The figure shows three views and two pictorial views of one solid part (mm, origin at its lowest corner). Answer the questions. A direction names the side the tool comes from. Coordinates: 2 decimals unless noted, no trailing zeros. Loops run counter-clockwise (first coordinate to the right, second up) from the corner with the lowest first, then second, coordinate; pieces in that order, holes last. Notation, with made-up numbers: (45.5, -11.75) -> (64.5, -11.75) arc R30 ccw to (64.5, 19.25) -> close; hole circle Ø1 at (43.5, -37.5). An arc over 180 degrees is marked (long way). Answer as a JSON object with one key per item and string values. Group by question number.
1) Determine the mould class of the marked faces 3, 4 and 5 for opening direction Y: released by +Y, released by -Y, zero draft, split by the parting line, or undercut.
2) Section C-C, the plane x = 3.5 is taken. Give the vertices of the cut face in (y, z).
3) Section A-A, the plane y = 6 is taken. Give the vertices of the cut face in (x, z).
4) Consider probe 1 along X at (y, z) = (5.75, 5.3); probe 2 along Y at (x, z) = (2.5, 1); probe 3 along X at (y, z) = (6.75, 5.3). Determine where each line is inside the solid, lowest interval first. Write a range as [from, to].
5) A flat-ended cylindrical pin translates along its axis: P1, Ø1.2, axis at x = 3.5, z = 1.5, coming from the +Y side. Find the tip coordinate at first contact, or state that the pin passes through.
6) Section D-D, the plane y = 7.75 is taken. Give the vertices of the cut face in (x, z), plus the area to 3 significant figures.
7) Which of the six approach directions +Z, -Z, +X, -X, +Y, -Y give full straight-line access (tool end or side, diameter ignored) to the marked faces 1 and 2?
8) Section B-B, the plane z = 1.7 is taken. Give the vertices of the cut face in (x, y).
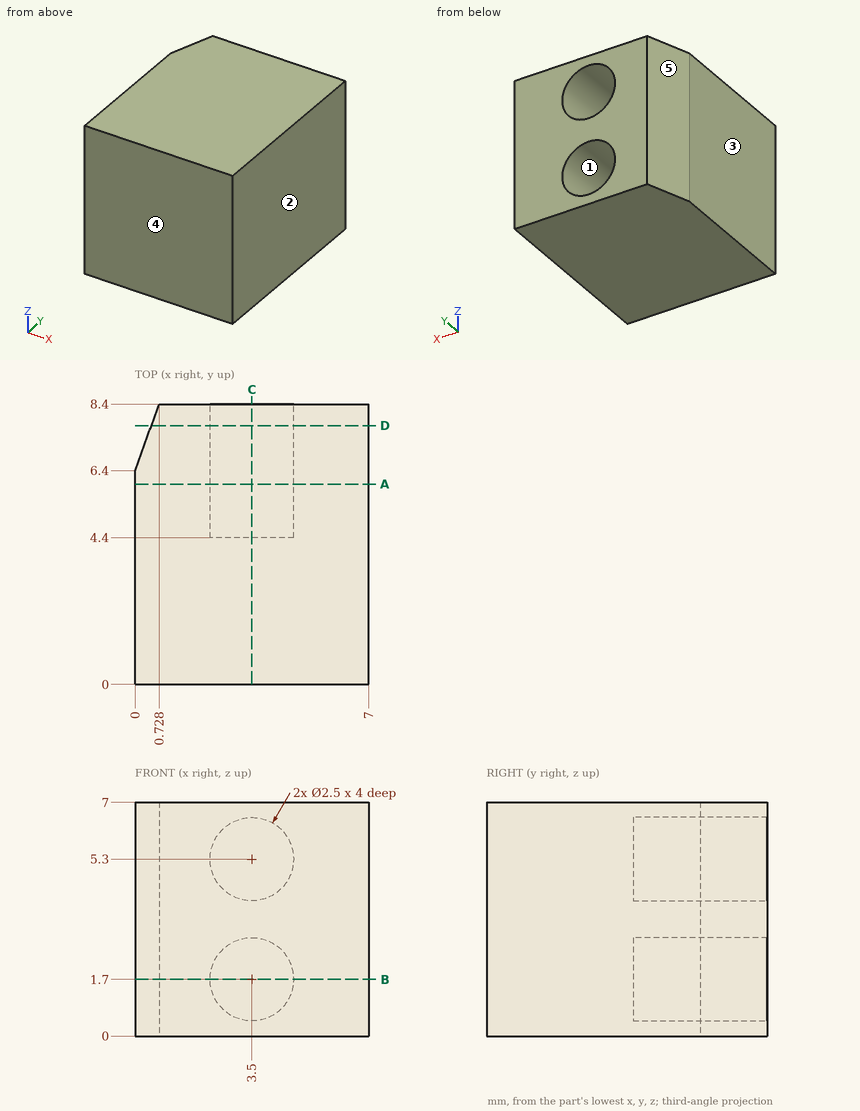
Determined:
{
 "1": {"face 3": "zero draft", "face 4": "released by -Y", "face 5": "released by +Y"},
 "2": {"outline": "(0, 0) -> (8.4, 0) -> (8.4, 0.45) -> (4.4, 0.45) -> (4.4, 2.95) -> (8.4, 2.95) -> (8.4, 4.05) -> (4.4, 4.05) -> (4.4, 6.55) -> (8.4, 6.55) -> (8.4, 7) -> (0, 7) -> close"},
 "3": {"outline": "(0, 0) -> (7, 0) -> (7, 7) -> (0, 7) -> close; hole circle Ø2.5 at (3.5, 1.7); hole circle Ø2.5 at (3.5, 5.3)"},
 "4": {"probe 1": "[0, 2.25], [4.75, 7]", "probe 2": "[0, 4.4]", "probe 3": "[0.13, 2.25], [4.75, 7]"},
 "5": {"P1": "y = 4.4"},
 "6": {"outline": "(0.49, 0) -> (7, 0) -> (7, 7) -> (0.49, 7) -> close; hole circle Ø2.5 at (3.5, 1.7); hole circle Ø2.5 at (3.5, 5.3)", "area": "35.7 mm²"},
 "7": {"face 1": "+Y", "face 2": "+Z, -Z, +X, +Y, -Y"},
 "8": {"outline": "(0, 0) -> (7, 0) -> (7, 8.4) -> (4.75, 8.4) -> (4.75, 4.4) -> (2.25, 4.4) -> (2.25, 8.4) -> (0.73, 8.4) -> (0, 6.4) -> close"}
}
